CAD build for the part. Positions are in the model's coordinates, mm. Face numbers are marked on the shaded views. A direction names the side the tool comes from. Give positions to 0.01 mm unless a question says otherwise; leave off trailing zeros. Loops run counter-clockwise (first coordinate to the right, second up) from the corner with the lowest first, then second, coordinate; pieces in that order, holes last. Notation, with made-up numbers: (57, 43) -> (70, 43) arc R21 cw to (70, 60) -> close; hole circle Ø7 at (-8, 4.25). An arc over 180 degrees is marked (long way). Write each question's results on one line, items separated by ' | '. Start each with the question number.
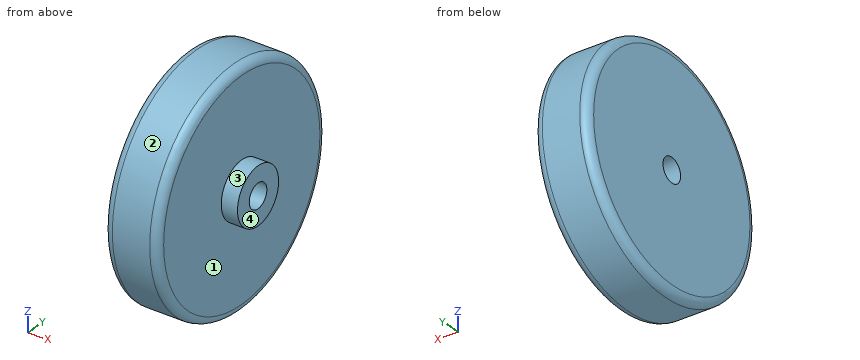
Autodesk Fusion 360 part; units mm, degrees
sketch "スケッチ1" plane through (0, 0, 0) normal (1, 0, 0) x (0, 0, -1)
  circle A0 centre (0, 0) radius 14.3
  dimension "d1" = 28.6
extrude "押し出し1" add sketch "スケッチ1" along normal blind 6.6
sketch "スケッチ2" plane through (6.6, 0, 0) normal (1, 0, 0) x (0, 0, -1)
  circle A0 centre (0, 0) radius 14.3
  circle A1 centre (0, 0) radius 3.5
  dimension "d4" = 7
extrude "押し出し2" add sketch "スケッチ2" along normal blind 2 contours A1
sketch "スケッチ3" plane through (8.6, 0, 0) normal (1, 0, 0) x (0, 0, -1)
  circle A0 centre (0, 0) radius 3.5
  circle A1 centre (0, 0) radius 1.5
  dimension "d7" = 3
extrude "押し出し3" cut sketch "スケッチ3" along normal mid plane 17.6 contours A1
fillet "フィレット1" radius 1 1 edges at (0, -5.1711, 13.3323)
fillet "フィレット2" radius 1 1 edges at (6.6, -5.1711, 13.3323)
Q1. Which spindle directions (+Z, -Z, +X, -X, +Y, -Y) get a long thin tool onto all of the face, cutting with end or side? Do the marked faces 3 and 4. Say none if no direction does.
Q2. Mould opens along Y. For the marked faces 1 and 2 say: pulls with the +Y half, pulls with the -Y half, needs draft (parallel to the pull), parting line crosses it, or undercut.
Q3. Saw through at C-C, the plane x = 4.75. List the corners of the cut face in (y, z), then the cut area to 3 significant figures.
Q4. Saw through at D-D, the plane x = 8.25. List the corners of the cut face in (y, z), then the cut area to 3 significant figures.
Q5. Drop flat-ended pins along their axis: pin 1 (1 mm diameter, centred on y = 11, z = -4, fed in from -X); pin 2 (6 mm diameter, centred on y = 8, z = -7, fed in from +X); pin 3 (1.5 mm diameter, centred on x = 4.5, z = -8.5, fed in from -Y); pin 4 (1.5 mm diameter, centred on x = 3, y = 4.5, fed in from -Z). Give the stop position or say it passes through.
Q6. Saw through at A-A, the plane y = 0. List the corners of the cut face in (x, z), then the cut area to 3 significant figures.
Q7. Wall check: L1, parallel to Y at x = 2.75, z = 0; L2, parallel to X at y = 5, z = 1.5; L3, parallel to Y at x = 5.5, z = 5.25. Give the ranges that are in metal, low to high.
Answer block:
1) face 3: +X | face 4: +Z, -Z, +X, +Y, -Y
2) face 1: needs draft | face 2: parting line crosses it
3) outline: circle Ø28.6 at (0, 0); hole circle Ø3 at (0, 0) | area: 635 mm2
4) outline: circle Ø7 at (0, 0); hole circle Ø3 at (0, 0) | area: 31.4 mm2
5) pin 1: stops at x = 0 | pin 2: stops at x = 6.6 | pin 3: stops at y = -12.02 | pin 4: stops at z = -13.8
6) outline: (0, -13.3) arc R1 ccw to (1, -14.3) -> (5.6, -14.3) arc R1 ccw to (6.6, -13.3) -> (6.6, -3.5) -> (8.6, -3.5) -> (8.6, -1.5) -> (0, -1.5) -> close; (0, 1.5) -> (8.6, 1.5) -> (8.6, 3.5) -> (6.6, 3.5) -> (6.6, 13.3) arc R1 ccw to (5.6, 14.3) -> (1, 14.3) arc R1 ccw to (0, 13.3) -> close | area: 176 mm2
7) L1: y = -14.3 to -1.5, 1.5 to 14.3 | L2: x = 0 to 6.6 | L3: y = -13.3 to 13.3
